Geometry check sheet. Reference: the model listing, model coordinates, mm. Face numbers are marked on the shaded views. A direction names the side the tool comes from. Coordinates: 2 decimals unless noted, no trailing zeros. Loops run counter-clockwise (first coordinate to the right, second up) from the corner with the lowest first, then second, coordinate; pieces in that order, holes last.
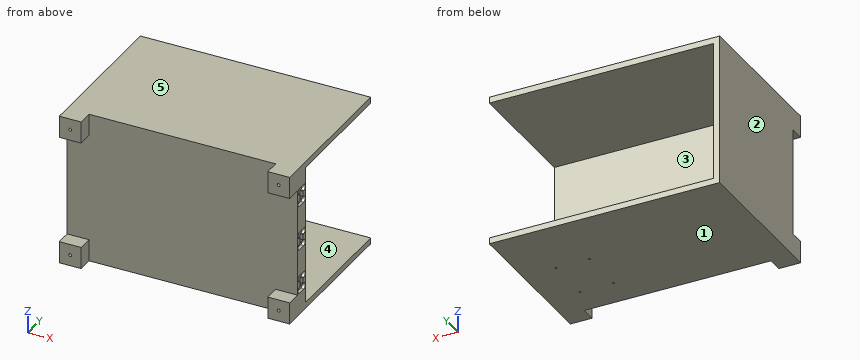
from build123d import *

# Parameters (mm, degrees)
SKETCH_1_W             = 380
SKETCH_1_H             = 250
EXTRUDE_1_DEPTH        = 233
SKETCH_4_W             = 36
SKETCH_4_H             = 36
EXTRUDE_2_DEPTH        = 25
HOLE_WIZARD_M6_1_D     = 5
HOLE_WIZARD_M6_1_DEPTH = 15
HOLE_WIZARD_M6_1_TIP   = 1.502151548
SKETCH_2_W             = 360
SKETCH_2_H             = 230
CUT_EXTRUDE_1_DEPTH    = 207
HOLE_WIZARD_M4_1_D     = 3.3
HOLE_WIZARD_M4_1_DEPTH = 10
SKETCH_7_W             = 10
SKETCH_7_H             = 230
CUT_EXTRUDE_3_DEPTH    = 207
HOLE_WIZARD_M2_1_D     = 1.6
HOLE_WIZARD_M2_1_DEPTH = 15
HOLE_WIZARD_M2_1_TIP   = 0.480688495
CUT_EXTRUDE_START      = -5
SKETCH_22_R            = 0.8
CUT_EXTRUDE_6_DEPTH    = 5


with BuildPart() as part:
    # 草图1 → 凸台-拉伸1 (new body)
    with BuildSketch(Plane(origin=(0, 0, 0), x_dir=(1, 0, 0), z_dir=(0, 1, 0))):
        with Locations((19.448818898, -32.543307087)):
            Rectangle(SKETCH_1_W, SKETCH_1_H)
    extrude(amount=EXTRUDE_1_DEPTH)

    # 草图4 → 凸台-拉伸2 (add)
    with BuildSketch(Plane.XZ):
        with Locations((-152.551181102, 139.543307087)):
            Rectangle(SKETCH_4_W, SKETCH_4_H)
        with Locations((191.448818898, 139.543307087)):
            Rectangle(SKETCH_4_W, SKETCH_4_H)
        with Locations((191.448818898, -74.456692913)):
            Rectangle(SKETCH_4_W, SKETCH_4_H)
        with Locations((-152.551181102, -74.456692913)):
            Rectangle(SKETCH_4_W, SKETCH_4_H)
    extrude(amount=EXTRUDE_2_DEPTH)

    # M6 螺纹孔1
    with Locations(Plane.XZ.offset(25)):
        with Locations((-152.551181102, -74.456692913), (-152.551181102, 139.543307087), (191.448818898, 139.543307087), (191.448818898, -74.456692913)):
            Hole(HOLE_WIZARD_M6_1_D / 2, depth=HOLE_WIZARD_M6_1_DEPTH)
            with Locations((0, 0, -(HOLE_WIZARD_M6_1_DEPTH + HOLE_WIZARD_M6_1_TIP / 2))):  # 118° drill point
                Cone(0, HOLE_WIZARD_M6_1_D / 2, HOLE_WIZARD_M6_1_TIP, mode=Mode.SUBTRACT)

    # 草图2 → 切除-拉伸1 (cut)
    with BuildSketch(Plane(origin=(0, 233, 0), x_dir=(1, 0, 0), z_dir=(0, 1, 0))):
        with Locations((19.448818898, -32.543307087)):
            Rectangle(SKETCH_2_W, SKETCH_2_H)
    extrude(amount=-CUT_EXTRUDE_1_DEPTH, mode=Mode.SUBTRACT)

    # M4 螺纹孔1
    with Locations(Plane(origin=(0, 0, -92.456692913), x_dir=(-1, 0, 0), z_dir=(0, 0, -1))):
        with Locations((-154.448818898, 127), (-99.448818898, 127), (-154.448818898, 50), (-99.448818898, 50)):
            Hole(HOLE_WIZARD_M4_1_D / 2, depth=HOLE_WIZARD_M4_1_DEPTH)

    # 草图7 → 切除-拉伸3 (cut)
    with BuildSketch(Plane(origin=(0, 233, 0), x_dir=(1, 0, 0), z_dir=(0, 1, 0))):
        with Locations((204.448818898, -32.543307087)):
            Rectangle(SKETCH_7_W, SKETCH_7_H)
    extrude(amount=-CUT_EXTRUDE_3_DEPTH, mode=Mode.SUBTRACT)

    # M2 螺纹孔1
    with Locations(Plane(origin=(209.448818898, 19.97945856, 116.543307087), x_dir=(0, 0, 1), z_dir=(1, 0, 0))):
        with Locations((0, 0), (0, 14), (-20, 14), (-20, 0), (-74, 0), (-74, 14), (-94, 0), (-94, 14), (-148, 0), (-168, 0), (-148, 14), (-168, 14)):
            Hole(HOLE_WIZARD_M2_1_D / 2, depth=HOLE_WIZARD_M2_1_DEPTH)
            with Locations((0, 0, -(HOLE_WIZARD_M2_1_DEPTH + HOLE_WIZARD_M2_1_TIP / 2))):  # 118° drill point
                Cone(0, HOLE_WIZARD_M2_1_D / 2, HOLE_WIZARD_M2_1_TIP, mode=Mode.SUBTRACT)

    # 草图22 → 切除-拉伸6 (cut)
    # profile 1 of 3: a face of its own
    with BuildSketch(Plane(origin=(209.448818898, 0, 0), x_dir=(0, 0, -1), z_dir=(1, 0, 0)).offset(CUT_EXTRUDE_START)):
        with BuildLine():
            Line((-101.543307087, 6.97945856), (-101.543307087, 5.97945856))
            ThreePointArc((-101.543307087, 5.97945856), (-96.543307087, 0.97945856), (-91.543307087, 5.97945856))
            Line((-91.543307087, 5.97945856), (-91.543307087, 19.97945856))
            ThreePointArc((-91.543307087, 19.97945856), (-96.543307087, 24.97945856), (-101.543307087, 19.97945856))
            Line((-101.543307087, 19.97945856), (-101.543307087, 18.97945856))
            ThreePointArc((-101.543307087, 18.97945856), (-101.836200305, 18.272351779), (-102.543307087, 17.97945856))
            Line((-102.543307087, 17.97945856), (-110.543307087, 17.97945856))
            ThreePointArc((-110.543307087, 17.97945856), (-111.250413868, 18.272351779), (-111.543307087, 18.97945856))
            Line((-111.543307087, 18.97945856), (-111.543307087, 19.97945856))
            ThreePointArc((-111.543307087, 19.97945856), (-116.543307087, 24.97945856), (-121.543307087, 19.97945856))
            Line((-121.543307087, 19.97945856), (-121.543307087, 5.97945856))
            ThreePointArc((-121.543307087, 5.97945856), (-116.543307087, 0.97945856), (-111.543307087, 5.97945856))
            Line((-111.543307087, 5.97945856), (-111.543307087, 6.97945856))
            ThreePointArc((-111.543307087, 6.97945856), (-111.250413868, 7.686565341), (-110.543307087, 7.97945856))
            Line((-110.543307087, 7.97945856), (-102.543307087, 7.97945856))
            ThreePointArc((-102.543307087, 7.97945856), (-101.836200305, 7.686565341), (-101.543307087, 6.97945856))
        make_face()
        with Locations((-96.543307087, 5.97945856)):
            Circle(SKETCH_22_R, mode=Mode.SUBTRACT)
        with Locations((-96.543307087, 19.97945856)):
            Circle(SKETCH_22_R, mode=Mode.SUBTRACT)
        with Locations((-116.543307087, 5.97945856)):
            Circle(SKETCH_22_R, mode=Mode.SUBTRACT)
        with Locations((-116.543307087, 19.97945856)):
            Circle(SKETCH_22_R, mode=Mode.SUBTRACT)
    # profile 2 of 3: a face of its own
    with BuildSketch(Plane(origin=(209.448818898, 0, 0), x_dir=(0, 0, -1), z_dir=(1, 0, 0)).offset(CUT_EXTRUDE_START)):
        with BuildLine():
            ThreePointArc((46.456692913, 5.97945856), (51.456692913, 0.97945856), (56.456692913, 5.97945856))
            Line((56.456692913, 5.97945856), (56.456692913, 19.97945856))
            ThreePointArc((56.456692913, 19.97945856), (51.456692913, 24.97945856), (46.456692913, 19.97945856))
            Line((46.456692913, 19.97945856), (46.456692913, 18.97945856))
            ThreePointArc((46.456692913, 18.97945856), (46.163799695, 18.272351779), (45.456692913, 17.97945856))
            Line((45.456692913, 17.97945856), (37.456692913, 17.97945856))
            ThreePointArc((37.456692913, 17.97945856), (36.749586132, 18.272351779), (36.456692913, 18.97945856))
            Line((36.456692913, 18.97945856), (36.456692913, 19.97945856))
            ThreePointArc((36.456692913, 19.97945856), (31.456692913, 24.97945856), (26.456692913, 19.97945856))
            Line((26.456692913, 19.97945856), (26.456692913, 5.97945856))
            ThreePointArc((26.456692913, 5.97945856), (31.456692913, 0.97945856), (36.456692913, 5.97945856))
            Line((36.456692913, 5.97945856), (36.456692913, 6.97945856))
            ThreePointArc((36.456692913, 6.97945856), (36.749586132, 7.686565341), (37.456692913, 7.97945856))
            Line((37.456692913, 7.97945856), (45.456692913, 7.97945856))
            ThreePointArc((45.456692913, 7.97945856), (46.163799695, 7.686565341), (46.456692913, 6.97945856))
            Line((46.456692913, 6.97945856), (46.456692913, 5.97945856))
        make_face()
        with Locations((31.456692913, 19.97945856)):
            Circle(SKETCH_22_R, mode=Mode.SUBTRACT)
        with Locations((31.456692913, 5.97945856)):
            Circle(SKETCH_22_R, mode=Mode.SUBTRACT)
        with Locations((51.456692913, 19.97945856)):
            Circle(SKETCH_22_R, mode=Mode.SUBTRACT)
        with Locations((51.456692913, 5.97945856)):
            Circle(SKETCH_22_R, mode=Mode.SUBTRACT)
    # profile 3 of 3: a face of its own
    with BuildSketch(Plane(origin=(209.448818898, 0, 0), x_dir=(0, 0, -1), z_dir=(1, 0, 0)).offset(CUT_EXTRUDE_START)):
        with BuildLine():
            Line((-27.543307087, 6.97945856), (-27.543307087, 5.97945856))
            ThreePointArc((-27.543307087, 5.97945856), (-22.543307087, 0.97945856), (-17.543307087, 5.97945856))
            Line((-17.543307087, 5.97945856), (-17.543307087, 19.97945856))
            ThreePointArc((-17.543307087, 19.97945856), (-22.543307087, 24.97945856), (-27.543307087, 19.97945856))
            Line((-27.543307087, 19.97945856), (-27.543307087, 18.97945856))
            ThreePointArc((-27.543307087, 18.97945856), (-27.836200305, 18.272351779), (-28.543307087, 17.97945856))
            Line((-28.543307087, 17.97945856), (-36.543307087, 17.97945856))
            ThreePointArc((-36.543307087, 17.97945856), (-37.250413868, 18.272351779), (-37.543307087, 18.97945856))
            Line((-37.543307087, 18.97945856), (-37.543307087, 19.97945856))
            ThreePointArc((-37.543307087, 19.97945856), (-42.543307087, 24.97945856), (-47.543307087, 19.97945856))
            Line((-47.543307087, 19.97945856), (-47.543307087, 5.97945856))
            ThreePointArc((-47.543307087, 5.97945856), (-42.543307087, 0.97945856), (-37.543307087, 5.97945856))
            Line((-37.543307087, 5.97945856), (-37.543307087, 6.97945856))
            ThreePointArc((-37.543307087, 6.97945856), (-37.250413868, 7.686565341), (-36.543307087, 7.97945856))
            Line((-36.543307087, 7.97945856), (-28.543307087, 7.97945856))
            ThreePointArc((-28.543307087, 7.97945856), (-27.836200305, 7.686565341), (-27.543307087, 6.97945856))
        make_face()
        with Locations((-42.543307087, 19.97945856)):
            Circle(SKETCH_22_R, mode=Mode.SUBTRACT)
        with Locations((-42.543307087, 5.97945856)):
            Circle(SKETCH_22_R, mode=Mode.SUBTRACT)
        with Locations((-22.543307087, 19.97945856)):
            Circle(SKETCH_22_R, mode=Mode.SUBTRACT)
        with Locations((-22.543307087, 5.97945856)):
            Circle(SKETCH_22_R, mode=Mode.SUBTRACT)
    extrude(amount=CUT_EXTRUDE_6_DEPTH, mode=Mode.SUBTRACT)


solid = part.part
(1) Sectioned sample at D-D on x = -144.5. Record the cut outline in (y, z), and give its area (3 significant figures).
Findings:
outline: (-25, -92.46) - (233, -92.46) - (233, -82.46) - (26, -82.46) - (26, 147.54) - (233, 147.54) - (233, 157.54) - (-25, 157.54) - (-25, 121.54) - (0, 121.54) - (0, -56.46) - (-25, -56.46) - close
area: 12,400 mm2
(2) Sectioned sample at B-B on y = 170.5. Record the cut outline in (x, z).
Findings:
outline: (-170.55, -92.46) - (209.45, -92.46) - (209.45, -82.46) - (-160.55, -82.46) - (-160.55, 147.54) - (209.45, 147.54) - (209.45, 157.54) - (-170.55, 157.54) - close
(3) Sectioned sample at A-A on x = 68. Record the cut outline in (y, z), and give its area (3 significant figures).
Findings:
outline: (0, -92.46) - (233, -92.46) - (233, -82.46) - (26, -82.46) - (26, 147.54) - (233, 147.54) - (233, 157.54) - (0, 157.54) - close
area: 10,600 mm2
(4) Gauge pin test, flat ends, axial feed: pin 1 Ø4.5 at (x, z) = (191.45, 139.54) entering from +Y; pin 2 Ø3 at (x, z) = (-152.55, 139.54) entering from -Y; pin 3 Ø1 at (y, z) = (5.98, -51.46) entering from +X. Record the tip position at first contact, or that the pin passes through.
Findings:
pin 1: stops at y = 26
pin 2: stops at y = -9.4
pin 3: stops at x = 194.27
(5) Sectioned sample at C-C on z = 75.5. Record the cut outline in (x, y), and give its area (4 significant figures).
Findings:
outline: (-170.55, 0) - (209.45, 0) - (209.45, 26) - (-160.55, 26) - (-160.55, 233) - (-170.55, 233) - close
area: 11,950 mm2
(6) Draft check along Z on the marked faces 1, 2 and 3. Enter one of: +Z half, -Z half, draft (parallel to the pull), parting line (faces both ways), or undercut.
Findings:
face 1: -Z half
face 2: draft
face 3: undercut
(7) Scan lines: L1, parallel to Z at x = 173, y = 70.5; L2, parallel to Y at x = 170.5, z = 60; L3, parallel to X at y = 185, z = 25. Record each from-to range of solid material in increasing order.
Findings:
L1: z = -92.46 to -82.46, 147.54 to 157.54
L2: y = 0 to 26
L3: x = -170.55 to -160.55
(8) Access from +Z, -Z, +X, -X, +Y, -Y to the whole of each face (thin tool, end or side, straight path). Record for the marked faces 4 and 5.
Findings:
face 4: +X, +Y
face 5: +Z, +X, -X, +Y, -Y
